Design review of the part built by this model. Coordinates are the model's own, in mm. Give positions to 0.01 mm unless a question says otherwise; leave off trailing zeros. Loops run counter-clockwise (first coordinate to the right, second up) from the corner with the lowest first, then second, coordinate; pieces in that order, holes last. Notation, with made-up numbers: M 63.5,-18.75 L 98.5,-18.75 A28 cw 98.5,-0.75 Z; hole C 70,-33.5 d4. An arc over 180 degrees is marked long. Use a Markdown table: item, result. Add a question column.
(1) Add section A-A, the plane y = 2.3. Give the boundary of the cut face in (x, z) (3 decimals), then the cut area to 3 significant figures.
(2) Add section B-B, the plane x = -237.5. Give the boundary of the cut face in (y, z).
(3) For probe 1 along Z at (x, y) = (-251.5, 1.5); probe 2 along X at (y, z) = (2.7, -37) (3 decimals), list the stretches that pass through material, from the lowest coordinate up.
(4) Insertion check: pin 1 Ø1.5 at (y, z) = (1, -27) entering from -X; pin 2 Ø1.5 at (x, z) = (-218.5, 5) entering from -Y; pin 3 Ø1.5 at (y, z) = (1.5, 43.5) entering from -X; pin 4 Ø0.9 at (y, z) = (1.5, 43) entering from +X. Each pin has a flat end and moves straight along its axis. Give the tip position at first contact, or say it passes through.
```python
from build123d import *

# Parameters (mm, degrees)
SKETCH1_W           = 630
SKETCH1_H           = 90
BOSS_EXTRUDE1_DEPTH = 3
SKETCH3_W           = 30
SKETCH3_H           = 3
CUT_EXTRUDE1_DEPTH  = 3
LPATTERN1_COUNT     = 10
LPATTERN1_PITCH     = 60
LPATTERN1_COL_COUNT = 2
LPATTERN1_COL_PITCH = 60
SKETCH7_W           = 3
SKETCH7_H           = 30
CUT_EXTRUDE3_DEPTH  = 3
SKETCH13_W          = 3
SKETCH13_H          = 27
CUT_EXTRUDE4_DEPTH  = 10


with BuildPart() as part:
    # Sketch1 → Boss-Extrude1 (new body)
    with BuildSketch(Plane(origin=(0, 0, 0), x_dir=(1, 0, 0), z_dir=(0, 1, 0))):
        Rectangle(SKETCH1_W, SKETCH1_H)
    extrude(amount=BOSS_EXTRUDE1_DEPTH)

    # Sketch3 → Cut-Extrude1 (cut)
    with BuildSketch(Plane(origin=(0, 3, 0), x_dir=(1, 0, 0), z_dir=(0, 1, 0))):
        with Locations((-240, -43.5)):
            Rectangle(SKETCH3_W, SKETCH3_H)
    cut_extrude1 = extrude(amount=-CUT_EXTRUDE1_DEPTH, mode=Mode.SUBTRACT)

    # LPattern1: Cut-Extrude1 ×10
    with Locations(*[(i * LPATTERN1_PITCH, 0, 0) for i in range(1, LPATTERN1_COUNT)]):
        add(cut_extrude1, mode=Mode.SUBTRACT)

    # LPattern1 col: Cut-Extrude1 ×2
    with Locations(*[(-i * LPATTERN1_COL_PITCH, 0, 0) for i in range(1, LPATTERN1_COL_COUNT)]):
        add(cut_extrude1, mode=Mode.SUBTRACT)

    # Sketch7 → Cut-Extrude3 (cut)
    with BuildSketch(Plane(origin=(0, 3, 0), x_dir=(1, 0, 0), z_dir=(0, 1, 0))):
        with Locations((-313.5, 30)):
            Rectangle(SKETCH7_W, SKETCH7_H)
    extrude(amount=-CUT_EXTRUDE3_DEPTH, mode=Mode.SUBTRACT)

    # Sketch13 → Cut-Extrude4 (cut)
    with BuildSketch(Plane(origin=(0, 3, 0), x_dir=(1, 0, 0), z_dir=(0, 1, 0))):
        with Locations((-313.5, -28.5)):
            Rectangle(SKETCH13_W, SKETCH13_H)
    extrude(amount=-CUT_EXTRUDE4_DEPTH, mode=Mode.SUBTRACT)

    # SurfaceCut1
    split(bisect_by=Plane(origin=(-0.725, 0, 0), x_dir=(0, 0, -1), z_dir=(1, 0, 0)), keep=Keep.BOTTOM)


solid = part.part
```
Established:
| question | item | result |
|---|---|---|
| 1 | outline | M -315,-15 L -312,-15 L -312,-45 L -0.725,-45 L -0.725,42 L -15,42 L -15,45 L -45,45 L -45,42 L -75,42 L -75,45 L -105,45 L -105,42 L -135,42 L -135,45 L -165,45 L -165,42 L -195,42 L -195,45 L -225,45 L -225,42 L -255,42 L -255,45 L -285,45 L -285,42 L -312,42 L -312,15 L -315,15 Z |
| 1 | area | 27,600 mm^2 |
| 2 | outline | M 0,-45 L 3,-45 L 3,42 L 0,42 Z |
| 3 | probe 1 | -45 to 42 |
| 3 | probe 2 | -312 to -0.725 |
| 4 | pin 1 | x = -312 |
| 4 | pin 2 | y = 0 |
| 4 | pin 3 | x = -285 |
| 4 | pin 4 | x = -15 |
